```python
from build123d import *

# Parameters (mm, degrees)
SKETCH1_W           = 300
SKETCH1_H           = 210
BOSS_EXTRUDE1_DEPTH = 5
SKETCH2_W           = 67.619836516
SKETCH2_H           = 30
SKETCH2_W_2         = 72.619836516
SKETCH2_W_3         = 53.212613818
CUT_EXTRUDE1_DEPTH  = 6


with BuildPart() as part:
    # Sketch1 → Boss-Extrude1 (new body)
    with BuildSketch(Plane.XY):
        Rectangle(SKETCH1_W, SKETCH1_H)
    extrude(amount=BOSS_EXTRUDE1_DEPTH)

    # Sketch2 → Cut-Extrude1 (cut, through all)
    with BuildSketch(Plane(origin=(0, 0, 0), x_dir=(-1, 0, 0), z_dir=(0, 0, -1))):
        with Locations((-178.809918258, 65)):
            Rectangle(SKETCH2_W, SKETCH2_H)
        with Locations((-181.309918258, 5)):
            Rectangle(SKETCH2_W_2, SKETCH2_H)
        with Locations((-181.309918258, -55)):
            Rectangle(SKETCH2_W_2, SKETCH2_H)
        with Locations((171.606306909, 65)):
            Rectangle(SKETCH2_W_3, SKETCH2_H)
        with Locations((181.309918258, 5)):
            Rectangle(SKETCH2_W_2, SKETCH2_H)
        with Locations((181.309918258, -55)):
            Rectangle(SKETCH2_W_2, SKETCH2_H)
    extrude(amount=-CUT_EXTRUDE1_DEPTH, mode=Mode.SUBTRACT)


solid = part.part
```
Here's how the part is built. I have some questions about the finished solid (model axes, mm). Coordinates: 2 decimals unless noted, no trailing zeros. Order: outer loops, then holes, each group sorted by start corner. A loop starts at its lowest first (then second) coordinate and runs counter-clockwise, first axis right, second up. Notation, with made-up numbers: (88, -27.5) -> (114, -27.5) arc R23 ccw to (114, -15.5) -> close; hole circle Ø5 at (89, 5). An arc over 180 degrees is marked (long way). Return JSON: item names as keys, results as strings.
1) If I drill on probe 1 along X at (y, z) = (19.5, 3.25), over which ranges is the centre line in solid material (lowest first)?
Conclusion:
{"probe 1": "x = -145 to 145"}
2) If we section it at A-A on y = -46: List the corners of the cut face in (x, z) for me, plus the area to 3 significant figures.
Conclusion:
{"outline": "(-145, 0) -> (145, 0) -> (145, 5) -> (-145, 5) -> close", "area": "1,450 mm²"}
3) I'm going to push flat-ended pins straight in: P1, Ø2, axis at x = 42, y = -21.5, coming from the -Z side; P2, Ø2.5, axis at y = 2.5, z = 3.5, coming from the -X side; P3, Ø2.5, axis at y = 6.5, z = 1.5, coming from the +X side. Where does each tip first touch, or does it pass through?
Conclusion:
{"P1": "stops at z = 0", "P2": "stops at x = -145", "P3": "stops at x = 145"}
